CAD build for the part. Positions are in the model's coordinates, mm. Face numbers are marked on the shaded views. Round coordinates to 2 decimals unless told otherwise and drop trailing zeros. Write each loop counter-clockwise with the first axis right and the second up, starting at its lowest first coordinate (ties: lowest second). Pieces come first, ordered by that corner, then holes. Notation, with made-up numbers: (56, 27.25) - (112, 27.25) arc R14 ccw to (112, 34.25) - close; hole circle Ø2 at (76.5, -23). An arc over 180 degrees is marked (long way). Answer in a Markdown table with one row per item.
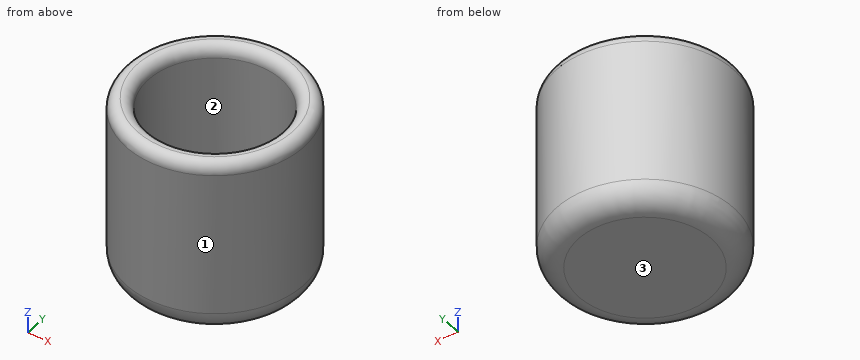
```python
from build123d import *

# Parameters (mm, degrees)
F0_R     = 25.4
F1_DEPTH = 50.8
F2_R     = 19.05
F3_DEPTH = 44.45
F4_R     = 3.17499
F5_R     = 12.7
F6_R     = 6.35


# Not quite as in the source:
# - a fillet or chamfer is up to 0.001 mm smaller than in the source, because OpenCascade refuses the exact size


with BuildPart() as f1:
    # F0 (on Top) → F1 (new body)
    with BuildSketch(Plane.XY):
        Circle(F0_R)
    extrude(amount=F1_DEPTH)

    # F2 (on face) → F3 (cut)
    with BuildSketch(Plane.XY.offset(50.8)):
        Circle(F2_R)
    extrude(amount=-F3_DEPTH, mode=Mode.SUBTRACT)

    # F4 (radius 3.175 in the source; OpenCascade refuses exactly that, so slightly less here)
    f4_edges = [f1.edges().sort_by_distance(p)[0] for p in [
        (-25.4, 0, 50.8),
        (-19.05, 0, 50.8),
    ]]
    fillet(f4_edges, radius=F4_R)

    # F5
    f5_edges = [f1.edges().sort_by_distance(p)[0] for p in [
        (-19.05, 0, 6.35),
    ]]
    fillet(f5_edges, radius=F5_R)

    # F6
    f6_edges = [f1.edges().sort_by_distance(p)[0] for p in [
        (-25.4, 0, 0),
    ]]
    fillet(f6_edges, radius=F6_R)


solid = f1.part
```
Q1. Saw through at A-A on z = 23.5. List the corners of the cut face in (x, y).
Computed:
| item | result |
|---|---|
| outline | circle Ø50.8 at (0, 0); hole circle Ø38.1 at (0, 0) |
Q2. Pull direction X, two halves, no side cores. Call the marked faces 1, 2 and 3: released by +X, released by -X, zero draft, split by the parting line, or undercut.
Computed:
| item | result |
|---|---|
| face 1 | split by the parting line |
| face 2 | undercut |
| face 3 | zero draft |
Q3. Drill centre lines: line 1 (Y direction, x = 0, z = 26); line 2 (X direction, y = 4, z = 49); line 3 (Y direction, x = -8.5, z = 21.5). Where is each one in solid material? Low to high.
Computed:
| item | result |
|---|---|
| line 1 | y = -25.4 to -19.05, 19.05 to 25.4 |
| line 2 | x = -24.77 to -18.95, 18.95 to 24.77 |
| line 3 | y = -23.94 to -17.05, 17.05 to 23.94 |
Q4. Flat gauge pins, fed straight in: pin 1 (1 mm diameter, centred on x = 11.5, y = -15.5, fed in from +Z); pin 2 (1 mm diameter, centred on x = -18.5, z = 34.5, fed in from +Y); pin 3 (1 mm diameter, centred on x = -8.5, z = 21.5, fed in from +Y). Where does each tip first touch, or does it go through?
Computed:
| item | result |
|---|---|
| pin 1 | stops at z = 49.67 |
| pin 2 | stops at y = 17.92 |
| pin 3 | stops at y = 24.11 |
